from build123d import *

# Parameters (mm, degrees)
CHAMFER1_SIZE = 1.25


with BuildPart() as part:
    # Sketch1 → Revolve1 (revolve)
    with BuildSketch(Plane.XY, mode=Mode.PRIVATE) as revolve1_sk:
        with BuildLine():
            Line((24.13, 3.81), (26.67, 1.27))
            Line((26.67, 1.27), (26.67, 0))
            Line((26.67, 0), (0, 0))
            Line((0, 0), (0, 76.02))
            Line((0, 76.02), (3.18, 76.02))
            Line((3.18, 76.02), (3.18, 19.06))
            ThreePointArc((3.18, 19.06), (7.646621587, 8.276621587), (18.43, 3.81))
            Line((18.43, 3.81), (24.13, 3.81))
        make_face()
    revolve(revolve1_sk.sketch.rotate(Axis((0, 76.02, 0), (0, -1, 0)), 180), axis=Axis((0, 76.02, 0), (0, -1, 0)))

    # Chamfer1
    chamfer1_edges = [part.edges().sort_by_distance(p)[0] for p in [
        (3.18, 76.02, 0),
    ]]
    chamfer(chamfer1_edges, length=CHAMFER1_SIZE)


solid = part.part
Input: part model. Units: mm. Frame: model coordinates. A direction names the side the tool comes from. Coordinates: 2 decimals unless noted, no trailing zeros. Loops run counter-clockwise (first coordinate to the right, second up) from the corner with the lowest first, then second, coordinate; pieces in that order, holes last.
Q1. Material intervals for line 1 (Y direction, x = -9, z = 19.5); line 2 (X direction, y = 28, z = 2); line 3 (Z direction, x = 0, y = 34), sorted ascending.
Q2. Contact query for flat-ended pins moving along their axis: pin 1 (4 mm diameter, centred on x = -8, z = 0.5, fed in from +Y); pin 2 (1 mm diameter, centred on x = 12.5, z = 6, fed in from +Y); pin 3 (12 mm diameter, centred on y = 20.5, z = 15, fed in from +X); pin 4 (8 mm diameter, centred on x = -18, z = -12, fed in from +Y). Output: stop coordinate, or through.
Q3. Cut plane B-B (z = 0). Output: boundary loops of the cut face in (x, y).
Q4. Cut plane A-A (x = 0). Output: boundary loops of the cut face in (y, z), then the cut area to 3 significant figures.
Q5. Cut plane C-C (y = 62). Output: boundary loops of the cut face in (x, z), then the cut area to 3 significant figures.
Q6. Cut plane D-D (y = 6). Output: boundary loops of the cut face in (x, z), then the cut area to 3 significant figures.
Q7. Set-up query: faces 1 (the face through (3.472, 0.626, -26.443)), 2 (the face through (-5, 3.81, 18)). Return all of +Z, -Z, +X, -X, +Y, -Y with unobstructed straight access to the full face (end or side cutting, diameter ignored); none if empty.
Working result:
1. line 1: y = 0 to 3.81
1. line 2: x = -2.47 to 2.47
1. line 3: z = -3.18 to 3.18
2. pin 1: stops at y = 10.2
2. pin 2: stops at y = 4.68
2. pin 3: passes through
2. pin 4: stops at y = 3.83
3. outline: (-26.67, 0) - (26.67, 0) - (26.67, 1.27) - (24.13, 3.81) - (18.43, 3.81) arc R15.25 cw to (3.18, 19.06) - (3.18, 74.77) - (1.93, 76.02) - (-1.93, 76.02) - (-3.18, 74.77) - (-3.18, 19.06) arc R15.25 cw to (-18.43, 3.81) - (-24.13, 3.81) - (-26.67, 1.27) - close
4. outline: (0, -26.67) - (1.27, -26.67) - (3.81, -24.13) - (3.81, -18.43) arc R15.25 cw to (19.06, -3.18) - (74.77, -3.18) - (76.02, -1.93) - (76.02, 1.93) - (74.77, 3.18) - (19.06, 3.18) arc R15.25 cw to (3.81, 18.43) - (3.81, 24.13) - (1.27, 26.67) - (0, 26.67) - close
4. area: 754 mm2
5. outline: circle Ø6.36 at (0, 0)
5. area: 31.8 mm2
6. outline: circle Ø21.11 at (0, 0)
6. area: 350 mm2
7. face 1: +Y, -Y
7. face 2: +Y
